from build123d import *

# Parameters (mm, degrees)
SKETCH1_W           = 2.9718
SKETCH1_H           = 6.35
SKETCH1_H_2         = 3.3782
SKETCH1_H_3         = 2.9718
SKETCH1_W_2         = 19.05
BOSS_EXTRUDE1_DEPTH = 2.9718
CUT_EXTRUDE1_DEPTH  = 3.9718


with BuildPart() as part:
    # Sketch1 → Boss-Extrude1 (new body)
    with BuildSketch(Plane.XY):
        Polygon((-31.75, -6.35), (-31.75, -9.7282), (-12.7, -9.7282), (12.7, -9.7282), (31.75, -9.7282), (31.75, -6.35), (31.75, 6.35), (31.75, 12.7), (-31.75, 12.7), (-31.75, 6.35), align=None)
        with Locations((-33.2359, 9.525)):
            Rectangle(SKETCH1_W, SKETCH1_H)
        with Locations((-33.2359, -8.0391)):
            Rectangle(SKETCH1_W, SKETCH1_H_2)
        with Locations((-33.2359, -11.2141)):
            Rectangle(SKETCH1_W, SKETCH1_H_3)
        with Locations((-22.225, -11.2141)):
            Rectangle(SKETCH1_W_2, SKETCH1_H_3)
        with Locations((22.225, -11.2141)):
            Rectangle(SKETCH1_W_2, SKETCH1_H_3)
        with Locations((33.2359, -8.0391)):
            Rectangle(SKETCH1_W, SKETCH1_H_2)
        with Locations((33.2359, -11.2141)):
            Rectangle(SKETCH1_W, SKETCH1_H_3)
        with Locations((33.2359, 9.525)):
            Rectangle(SKETCH1_W, SKETCH1_H)
    extrude(amount=BOSS_EXTRUDE1_DEPTH)

    # Sketch2 → Cut-Extrude1 (cut, through all)
    with BuildSketch(Plane.XY.offset(2.9718)):
        Polygon((-20.7518, 3.175), (-20.7518, -3.175), (-23.2918, -3.175), (-23.2918, -1.524), (-31.75, -1.524), (-31.75, 1.524), (-23.2918, 1.524), (-23.2918, 3.175), align=None)
        Polygon((-3.175, 1.27), (3.175, 1.27), (3.175, -1.27), (1.524, -1.27), (1.524, -9.7282), (-1.524, -9.7282), (-1.524, -1.27), (-3.175, -1.27), align=None)
        Polygon((20.7518, 3.175), (20.7518, -3.175), (23.2918, -3.175), (23.2918, -1.524), (31.75, -1.524), (31.75, 1.524), (23.2918, 1.524), (23.2918, 3.175), align=None)
    extrude(amount=-CUT_EXTRUDE1_DEPTH, mode=Mode.SUBTRACT)


solid = part.part
Input: part model. Units: mm. Frame: model coordinates. A direction names the side the tool comes from. Round coordinates to 2 decimals unless told otherwise and drop trailing zeros. Order: outer loops, then holes, each group sorted by start corner. A loop starts at its lowest first (then second) coordinate and runs counter-clockwise, first axis right, second up. Notation, with made-up numbers: (14, 51) - (37, 51) arc R22 cw to (37, 84) - close; hole circle Ø3 at (-10.75, 26.5). An arc over 180 degrees is marked (long way). Use a Markdown table: item, result.
1. Access query for faces 4 (the face through (33, 6.35, 1)), 5 (the face through (-31.75, 4, 1)), 6 (the face through (23.292, 2, 2)). Directions: +Z, -Z, +X, -X, +Y, -Y. A direction counts if a zero-diameter tool reaches every point of the face in a straight line with its end or side. Return the directions, or none.
Evaluation:
| item | result |
|---|---|
| face 4 | +Z, -Z, +X |
| face 5 | +Z, -Z, -X |
| face 6 | +Z, -Z |
2. Mould query, pull axis Y, two halves, no side actions, for faces 1 (the face through (24, -12.7, 1)), 2 (the face through (-27, -1.524, 2)), 3 (the face through (-34.722, -9, 1)). Classes: +Y half, -Y half, draft (parallel to the pull), parting line (faces both ways), or undercut.
Evaluation:
| item | result |
|---|---|
| face 1 | -Y half |
| face 2 | undercut |
| face 3 | draft |
3. Section A-A on x = -29. Return the cut outline in (y, z).
Evaluation:
| item | result |
|---|---|
| outline | (-12.7, 0) - (-1.52, 0) - (-1.52, 2.97) - (-12.7, 2.97) - close; (1.52, 0) - (12.7, 0) - (12.7, 2.97) - (1.52, 2.97) - close |
4. Section B-B on x = -6. Return the cut outline in (y, z), then the cut area to 3 significant figures.
Evaluation:
| item | result |
|---|---|
| outline | (-9.73, 0) - (12.7, 0) - (12.7, 2.97) - (-9.73, 2.97) - close |
| area | 66.7 mm^2 |
5. First-contact query: pin 1 (0.8 mm diameter, centred on y = 2.5, z = 1, fed in from -X); pin 2 (0.8 mm diameter, centred on y = -0.5, z = 1.5, fed in from +X); pin 3 (1.3 mm diameter, centred on y = 2.5, z = 2, fed in from +X). Flat tips, straight axial feed; report the tip coordinate or a pass-through.
Evaluation:
| item | result |
|---|---|
| pin 1 | x = -31.75 |
| pin 2 | x = 20.75 |
| pin 3 | x = 31.75 |
6. Material intervals for probe 1 along X at (y, z) = (2, 2.5); probe 2 along Y at (x, z) = (31.5, 2.5); probe 3 along X at (y, z) = (-5, 1.5), sorted ascending.
Evaluation:
| item | result |
|---|---|
| probe 1 | -31.75 to -23.29, -20.75 to 20.75, 23.29 to 31.75 |
| probe 2 | -12.7 to -1.52, 1.52 to 12.7 |
| probe 3 | -31.75 to -1.52, 1.52 to 31.75 |
